from build123d import *

# Parameters (mm, degrees)
BOSS_EXTRUDE1_DEPTH  = 25
BOSS_EXTRUDE2_DEPTH  = 2
SKETCH3_W            = 72.5
SKETCH3_H            = 18.058244084
CUT_EXTRUDE1_DEPTH   = 90
SKETCH4_R            = 3.5
BOSS_EXTRUDE9_DEPTH  = 28.5
SKETCH5_R            = 1.5
CUT_EXTRUDE2_DEPTH   = 28.5
SKETCH6_R            = 3
CUT_EXTRUDE3_DEPTH   = 27
SKETCH7_W            = 70
SKETCH7_H            = 62
CUT_EXTRUDE4_DEPTH   = 0.1
SKETCH8_W            = 76
SKETCH8_H            = 17
CUT_EXTRUDE5_DEPTH   = 0.1
FILLET1_R            = 2
CUT_EXTRUDE6_DEPTH   = 5
FILLET1_OF_MIRROR1_R = 2


with BuildPart() as part:
    # Sketch1 → Boss-Extrude1 (new body)
    with BuildSketch(Plane(origin=(0, 0, 0), x_dir=(1, 0, 0), z_dir=(0, 1, 0))):
        Polygon((-48, 45.25), (-36.25, 45.25), (-36.25, 34.75), (36.25, 34.75), (36.25, 45.25), (48, 45.25), (48, -45.25), (36.25, -45.25), (36.25, -34.75), (-36.25, -34.75), (-36.25, -45.25), (-48, -45.25), align=None)
        Polygon((-46, 43.25), (-38.25, 43.25), (-38.25, 32.75), (38.25, 32.75), (38.25, 43.25), (46, 43.25), (46, -43.25), (38.25, -43.25), (38.25, -32.75), (-38.25, -32.75), (-38.25, -43.25), (-46, -43.25), align=None, mode=Mode.SUBTRACT)
    extrude(amount=BOSS_EXTRUDE1_DEPTH)

    # Sketch2 → Boss-Extrude2 (add)
    with BuildSketch(Plane(origin=(0, 25, 0), x_dir=(1, 0, 0), z_dir=(0, 1, 0))):
        Polygon((36.25, -45.25), (48, -45.25), (48, 45.25), (36.25, 45.25), (36.25, 34.75), (-36.25, 34.75), (-36.25, 45.25), (-48, 45.25), (-48, -45.25), (-36.25, -45.25), (-36.25, -34.75), (36.25, -34.75), align=None)
    extrude(amount=BOSS_EXTRUDE2_DEPTH)

    # Sketch3 → Cut-Extrude1 (cut)
    with BuildSketch(Plane.XY.offset(34.75)):
        with Locations((0, 2.970877958)):
            Rectangle(SKETCH3_W, SKETCH3_H)
    extrude(amount=-CUT_EXTRUDE1_DEPTH, mode=Mode.SUBTRACT)

    # Sketch4 → Boss-Extrude9 (add)
    with BuildSketch(Plane(origin=(0, 27, 0), x_dir=(1, 0, 0), z_dir=(0, 1, 0))):
        with Locations(Location((-42.75, 40.25, 0), (0, 0, 270))):
            Circle(SKETCH4_R)
        with Locations(Location((42.75, 40.25, 0), (0, 0, 270))):
            Circle(SKETCH4_R)
        with Locations(Location((42.75, -40.25, 0), (0, 0, 270))):
            Circle(SKETCH4_R)
        with Locations(Location((-42.75, -40.25, 0), (0, 0, 270))):
            Circle(SKETCH4_R)
    extrude(amount=-BOSS_EXTRUDE9_DEPTH)

    # Sketch5 → Cut-Extrude2 (cut)
    with BuildSketch(Plane.XZ.offset(1.5)):
        with Locations(Location((-42.75, 40.25, 0), (0, 0, 270))):
            Circle(SKETCH5_R)
        with Locations(Location((42.75, 40.25, 0), (0, 0, 270))):
            Circle(SKETCH5_R)
        with Locations(Location((42.75, -40.25, 0), (0, 0, 270))):
            Circle(SKETCH5_R)
        with Locations(Location((-42.75, -40.25, 0), (0, 0, 270))):
            Circle(SKETCH5_R)
    extrude(amount=-CUT_EXTRUDE2_DEPTH, mode=Mode.SUBTRACT)

    # Sketch6 → Cut-Extrude3 (cut)
    with BuildSketch(Plane(origin=(0, 27, 0), x_dir=(1, 0, 0), z_dir=(0, 1, 0))):
        with Locations(Location((-42.75, 40.25, 0), (0, 0, 270))):
            Circle(SKETCH6_R)
        with Locations(Location((42.75, 40.25, 0), (0, 0, 90))):
            Circle(SKETCH6_R)
        with Locations(Location((42.75, -40.25, 0), (0, 0, 270))):
            Circle(SKETCH6_R)
        with Locations(Location((-42.75, -40.25, 0), (0, 0, 90))):
            Circle(SKETCH6_R)
    extrude(amount=-CUT_EXTRUDE3_DEPTH, mode=Mode.SUBTRACT)

    # Sketch7 → Cut-Extrude4 (cut)
    with BuildSketch(Plane(origin=(0, 27, 0), x_dir=(1, 0, 0), z_dir=(0, 1, 0))):
        Rectangle(SKETCH7_W, SKETCH7_H)
    extrude(amount=-CUT_EXTRUDE4_DEPTH, mode=Mode.SUBTRACT)

    # Sketch8 → Cut-Extrude5 (cut)
    with BuildSketch(Plane.ZY.offset(48)):
        with Locations((0, 12.5)):
            Rectangle(SKETCH8_W, SKETCH8_H)
    cut_extrude5 = extrude(amount=-CUT_EXTRUDE5_DEPTH, mode=Mode.SUBTRACT)

    # Fillet1
    fillet1_edges = [part.edges().sort_by_distance(p)[0] for p in [
        (-47.95, 21, 38),
        (-47.95, 4, 38),
        (-47.95, 4, -38),
        (-47.95, 21, -38),
    ]]
    fillet(fillet1_edges, radius=FILLET1_R)

    # Sketch9 → Cut-Extrude6 (cut)
    with BuildSketch(Plane.ZY.offset(47.9)):
        with BuildLine():
            Line((-34, 13.5), (-4, 13.5))
            ThreePointArc((-4, 13.5), (-3, 12.5), (-4, 11.5))
            Line((-4, 11.5), (-34, 11.5))
            ThreePointArc((-34, 11.5), (-35, 12.5), (-34, 13.5))
        make_face()
        with BuildLine():
            Line((-34, 17.5), (-4, 17.5))
            ThreePointArc((-4, 17.5), (-3, 16.5), (-4, 15.5))
            Line((-4, 15.5), (-34, 15.5))
            ThreePointArc((-34, 15.5), (-35, 16.5), (-34, 17.5))
        make_face()
        with BuildLine():
            Line((-34, 9.5), (-4, 9.5))
            ThreePointArc((-4, 9.5), (-3, 8.5), (-4, 7.5))
            Line((-4, 7.5), (-34, 7.5))
            ThreePointArc((-34, 7.5), (-35, 8.5), (-34, 9.5))
        make_face()
        with BuildLine():
            Line((34, 9.5), (4, 9.5))
            ThreePointArc((4, 9.5), (3, 8.5), (4, 7.5))
            Line((4, 7.5), (34, 7.5))
            ThreePointArc((34, 7.5), (35, 8.5), (34, 9.5))
        make_face()
        with BuildLine():
            Line((34, 13.5), (4, 13.5))
            ThreePointArc((4, 13.5), (3, 12.5), (4, 11.5))
            Line((4, 11.5), (34, 11.5))
            ThreePointArc((34, 11.5), (35, 12.5), (34, 13.5))
        make_face()
        with BuildLine():
            Line((34, 17.5), (4, 17.5))
            ThreePointArc((4, 17.5), (3, 16.5), (4, 15.5))
            Line((4, 15.5), (34, 15.5))
            ThreePointArc((34, 15.5), (35, 16.5), (34, 17.5))
        make_face()
    cut_extrude6 = extrude(amount=-CUT_EXTRUDE6_DEPTH, mode=Mode.SUBTRACT)

    # Mirror1: Cut-Extrude5, Cut-Extrude6 across plane
    add(cut_extrude5.mirror(Plane(origin=(0, 0, 0), x_dir=(0, 0, 1), z_dir=(1, 0, 0))), mode=Mode.SUBTRACT)
    add(cut_extrude6.mirror(Plane(origin=(0, 0, 0), x_dir=(0, 0, 1), z_dir=(1, 0, 0))), mode=Mode.SUBTRACT)

    # Fillet1 of Mirror1
    fillet1_of_mirror1_edges = [part.edges().sort_by_distance(p)[0] for p in [
        (47.95, 21, 38),
        (47.95, 4, 38),
        (47.95, 4, -38),
        (47.95, 21, -38),
    ]]
    fillet(fillet1_of_mirror1_edges, radius=FILLET1_OF_MIRROR1_R)


solid = part.part
Source: CAD feature listing. Evaluate the final solid. Frame: model axes, mm. A direction names the side the tool comes from. Round coordinates to 2 decimals unless told otherwise and drop trailing zeros. Loops run counter-clockwise (first coordinate to the right, second up) from the corner with the lowest first, then second, coordinate; pieces in that order, holes last. Notation, with made-up numbers: (85.5, -7) - (138.5, -7) arc R19 ccw to (138.5, 26) - close; hole circle Ø9 at (74.5, -18). An arc over 180 degrees is marked (long way). Write item = value, one per line. Start each with the question number.
(1) Pull-direction query (X, two-part tool) for faces 1 (the face through (-44.78, 13.69, 42.46)), 2 (the face through (-42, 13, -45.25)); classes: +X half, -X half, draft (parallel to the pull), parting line (faces both ways), or undercut.
(2) Ray query, line 1 along X through (y, z) = (8.5, 40.25); line 2 along X through (y, z) = (-0.35, 40.25); line 3 along X through (y, z) = (23.25, 36). Return the intervals inside material, ascending. Write a range as from..to.
(3) Pin query (flat end, axial travel): pin 1 (4 mm diameter, centred on y = 20, z = -3.5, fed in from -X); pin 2 (8 mm diameter, centred on x = 23, z = 16.5, fed in from -Y); pin 3 (4 mm diameter, centred on x = 3, z = 0, fed in from +Y); pin 4 (10 mm diameter, centred on y = 13.5, z = -2.5, fed in from -X). Return the tip coordinate at first contact, or that it passes through.
(4) Set-up query: faces 3 (the face through (1, 18, 32.75)), 4 (the face through (-42, 0, 42)), 5 (the face through (41, -1.5, 40)). Return all of +Z, -Z, +X, -X, +Y, -Y with unobstructed straight access to the full face (end or side cutting, diameter ignored); none if empty.
(5) Section query A-A, the plane x = -42.75. Output: boundary loops of the cut face in (y, z), plus the area to 3 significant figures.
(6) Section query C-C, the plane x = -9.5. Output: boundary loops of the cut face in (y, z).
(7) Section query B-B, the plane y = 2. State how many separate pieces and enclosed holes the cut face has, plus the area to 3 significant figures.
Conclusion:
q1.face_1 = undercut
q1.face_2 = draft
q2.line_1 = -48..-45.75, -39.75..-39.25, -38.25..-36.25, 36.25..38.25, 39.25..39.75, 45.75..48
q2.line_2 = -46.25..-44.25, -41.25..-39.25, 39.25..41.25, 44.25..46.25
q2.line_3 = -48..-46, -38.25..-36.25, 36.25..38.25, 46..48
q3.pin_1 = -48
q3.pin_2 = 25
q3.pin_3 = 26.9
q3.pin_4 = -47.9
q4.face_3 = -Y
q4.face_4 = +Y
q4.face_5 = +Z, -Z, +X, -X, -Y
q5.outline = (-1.5, -43.75) - (0, -43.75) - (0, -45.25) - (27, -45.25) - (27, -43.25) - (0, -43.25) - (0, -41.75) - (-1.5, -41.75) - close; (-1.5, -38.75) - (0, -38.75) - (0, -37.25) - (27, -37.25) - (27, 37.25) - (0, 37.25) - (0, 38.75) - (-1.5, 38.75) - (-1.5, 36.75) - (25, 36.75) - (25, -36.75) - (-1.5, -36.75) - close; (-1.5, 41.75) - (0, 41.75) - (0, 43.25) - (27, 43.25) - (27, 45.25) - (0, 45.25) - (0, 43.75) - (-1.5, 43.75) - close
q5.area = 294 mm2
q6.outline = (12, -34.75) - (27, -34.75) - (27, -31) - (26.9, -31) - (26.9, 31) - (27, 31) - (27, 34.75) - (12, 34.75) - (12, 32.75) - (25, 32.75) - (25, -32.75) - (12, -32.75) - close
q7.separate_pieces = 2
q7.enclosed_holes = 8
q7.area = 558 mm2
